```python
from build123d import *

# Parameters (mm, degrees)
F0_R     = 12.7
F1_DEPTH = 50.8
F2_SIZE  = 1.5875
F3_W     = 0.762
F3_H     = 1.8157000701
F6_R     = 0.127
F7_R     = 10.31875
F8_DEPTH = 50.801


with BuildPart() as f1:
    # F0 (on Front) → F1 (new body)
    with BuildSketch(Plane.XZ):
        Circle(F0_R)
    extrude(amount=F1_DEPTH)

    # F2
    f2_edges = [f1.edges().sort_by_distance(p)[0] for p in [
        (-12.7, -50.8, 0),
        (-12.7, 0, 0),
    ]]
    chamfer(f2_edges, length=F2_SIZE)

    # F3 (on Right) → F5 (revolve, cut)
    with BuildSketch(Plane.YZ):
        with Locations((-45.5422, 12.845850035)):
            Rectangle(F3_W, F3_H)
        with Locations((-5.2578, 12.845850035)):
            Rectangle(F3_W, F3_H)
    revolve(axis=Axis((0, -27.9251299798, 0), (0, -1, 0)), mode=Mode.SUBTRACT)

    # F6
    f6_edges = [f1.edges().sort_by_distance(p)[0] for p in [
        (-12.7, -49.2125, 0),
    ]]
    fillet(f6_edges, radius=F6_R)

    # F7 (on face) → F8 (cut, through all)
    with BuildSketch(Plane.XZ.offset(50.8)):
        Circle(F7_R)
    extrude(amount=-F8_DEPTH, mode=Mode.SUBTRACT)


solid = f1.part
```
Verification items for the finished model (mm, model axes). A direction names the side the tool comes from. Give positions to 0.01 mm unless a question says otherwise; leave off trailing zeros. Write each loop counter-clockwise with the first axis right and the second up, starting at its lowest first coordinate (ties: lowest second). Pieces come first, ordered by that corner, then holes. Notation, with made-up numbers: (32.5, -18) - (76.5, -18) arc R20 cw to (76.5, 3) - close; hole circle Ø6 at (-18.75, -19). An arc over 180 degrees is marked (long way). Put each result on its own line as item: value.
Q1. Set-up check for faces 1 (the face through (11.654, -5.252, -2.588)), 2 (the face through (-2.75, -25.12, -12.4)): record each of +Z, -Z, +X, -X, +Y, -Y from which the full face is reachable in a straight line by a thin tool's end or side.
Result:
face 1: none
face 2: +Y, -Y
Q2. Depth check by flat-ended pin: P1, Ø1, axis at x = -10, y = -39, coming from the +Z side; P2, Ø5, axis at y = -28.5, z = -9.5, coming from the -X side; P3, Ø8, axis at y = -38, z = 10, coming from the -X side; P4, Ø4, axis at x = -8, z = -1.5, coming from the -Y side. Enter the tip coordinate at first touch or a pass-through.
Result:
P1: z = 8.43
P2: x = -10.6
P3: x = -11.19
P4: through
Q3. Section check A-A on y = -21. Record the cut outline in (x, z), and give its area (3 significant figures).
Result:
outline: circle Ø25.4 at (0, 0); hole circle Ø20.64 at (0, 0)
area: 172 mm2
Q4. Mould release check, pull along X, two halves, no side actions. Record for faces 3 (the face through (4.6, -5.639, -11.2)), 4 (the face through (11.654, -45.537, -2.588)), 5 (the face through (-2.237, -25.756, -10.073)): released by +X, released by -X, zero draft, split by the parting line, or undercut.
Result:
face 3: zero draft
face 4: split by the parting line
face 5: undercut
Q5. Scan lines: probe 1 along Z at (x, y) = (0, -19); probe 2 along X at (y, z) = (-31.5, 3.5); probe 3 along X at (y, z) = (-12, 6.5). Record each from-to range of solid material in increasing order. Write a range as from..to.
Result:
probe 1: -12.7..-10.32, 10.32..12.7
probe 2: -12.21..-9.71, 9.71..12.21
probe 3: -10.91..-8.01, 8.01..10.91
